The model under review builds one solid part; all positions refer to its coordinate system, in mm. A direction names the side the tool comes from. Give positions to 0.01 mm unless a question says otherwise; leave off trailing zeros. Order: outer loops, then holes, each group sorted by start corner. A loop starts at its lowest first (then second) coordinate and runs counter-clockwise, first axis right, second up. Notation, with made-up numbers: M 83,81 L 133,81 A23 ccw 133,93 Z; hole C 81.5,-4.75 d9. An arc over 180 degrees is marked long. One line per question, with ' | ' between items. Start each with the question number.
1. Wall thickness on L1, parallel to X at y = 9.5, z = -39; L2, parallel to Y at x = 36.5, z = -43.5; L3, parallel to X at y = 38, z = -23: over which ranges is each line inside the solid? List them lowest first.
2. We need section D-D on x = 38. Write out the cut boundary in (y, z), then the cut area to 3 significant figures.
3. Insertion check: P1, Ø10, axis at x = 13.5, y = 11, coming from the -Z side; P2, Ø8, axis at x = 14.5, y = 16, coming from the +Z side. Each pin has a flat end and moves straight along its axis. Give the tip position at first contact, or say it passes through.
4. We need section B-B on x = 23.5. Write out the cut boundary in (y, z).
5. The part is to be moulded in two halves that separate along X. For faces 4 (the face through (37.03, 18.24, -37.08)), 5 (the face through (9.92, 18.24, -37.03)), 6 (the face through (45.2, 20.7, -1.7)), 7 (the face through (18, 42, -34)), say which applies: +X half, -X half, draft (parallel to the pull), parting line (faces both ways), or undercut.
6. For faces 1 (the face through (23, 2, -8)), 2 (the face through (35.111, 21, -41)), 3 (the face through (37.65, 20.78, -44.54)), list the 3-axis set-ups (+Z, -Z, +X, -X, +Y, -Y) from which the entire face can be reached by the end or side of a thin tool; tool diameter is ignored.
7. We need section C-C on z = -23.5. Write out the cut boundary in (x, y).
8. We need section A-A on y = 27. Write out the cut boundary in (x, z), then the cut area to 3 significant figures.
```python
from build123d import *

# Parameters (mm, degrees)
SKETCH1_R           = 1.75
SKETCH1_W           = 8
SKETCH1_H           = 23.221825406
SKETCH1_W_2         = 23.221825406
SKETCH1_H_2         = 8
BOSS_EXTRUDE1_DEPTH = 5
SKETCH1_3_R         = 1.75
SKETCH1_3_W         = 8
SKETCH1_3_H         = 23.221825406
BOSS_EXTRUDE2_DEPTH = 42
BOSS_EXTRUDE3_START = 37
SKETCH1_4_R         = 11.5
SKETCH1_4_W         = 23.221825406
SKETCH1_4_H         = 8
SKETCH1_4_R_2       = 1.75
SKETCH1_4_W_2       = 8
SKETCH1_4_H_2       = 23.221825406
BOSS_EXTRUDE3_DEPTH = 5
CHAMFER2_SIZE       = 5
CHAMFER4_SIZE       = 3.5


with BuildPart() as part:
    # Sketch1 → Boss-Extrude1 (new body)
    # profile 1 of 8: a face of its own
    with BuildSketch(Plane(origin=(0, 0, 0), x_dir=(1, 0, 0), z_dir=(0, 1, 0))):
        Polygon((0, 47), (0, 35.110912703), (8, 35.110912703), (11.889087297, 39), (11.889087297, 47), align=None)
        with Locations(Location((8, 39, 0), (0, 0, 270))):
            Circle(SKETCH1_R, mode=Mode.SUBTRACT)
    # profile 2 of 8: a face of its own
    with BuildSketch(Plane(origin=(0, 0, 0), x_dir=(1, 0, 0), z_dir=(0, 1, 0))):
        with Locations((4, 23.5)):
            Rectangle(SKETCH1_W, SKETCH1_H)
    # profile 3 of 8: a face of its own
    with BuildSketch(Plane(origin=(0, 0, 0), x_dir=(1, 0, 0), z_dir=(0, 1, 0))):
        Polygon((0, 11.889087297), (0, 0), (11.889087297, 0), (11.889087297, 8), (8, 11.889087297), align=None)
        with Locations(Location((8, 8, 0), (0, 0, 270))):
            Circle(SKETCH1_R, mode=Mode.SUBTRACT)
    # profile 4 of 8: a face of its own
    with BuildSketch(Plane(origin=(0, 0, 0), x_dir=(1, 0, 0), z_dir=(0, 1, 0))):
        with Locations((23.5, 4)):
            Rectangle(SKETCH1_W_2, SKETCH1_H_2)
    # profile 5 of 8: a face of its own
    with BuildSketch(Plane(origin=(0, 0, 0), x_dir=(1, 0, 0), z_dir=(0, 1, 0))):
        Polygon((35.110912703, 8), (35.110912703, 0), (47, 0), (47, 11.889087297), (39, 11.889087297), align=None)
        with Locations(Location((39, 8, 0), (0, 0, 270))):
            Circle(SKETCH1_R, mode=Mode.SUBTRACT)
    # profile 6 of 8: a face of its own
    with BuildSketch(Plane(origin=(0, 0, 0), x_dir=(1, 0, 0), z_dir=(0, 1, 0))):
        with Locations((43, 23.5)):
            Rectangle(SKETCH1_W, SKETCH1_H)
    # profile 7 of 8: a face of its own
    with BuildSketch(Plane(origin=(0, 0, 0), x_dir=(1, 0, 0), z_dir=(0, 1, 0))):
        Polygon((39, 35.110912703), (47, 35.110912703), (47, 47), (35.110912703, 47), (35.110912703, 39), align=None)
        with Locations(Location((39, 39, 0), (0, 0, 270))):
            Circle(SKETCH1_R, mode=Mode.SUBTRACT)
    # profile 8 of 8: a face of its own
    with BuildSketch(Plane(origin=(0, 0, 0), x_dir=(1, 0, 0), z_dir=(0, 1, 0))):
        with Locations((23.5, 43)):
            Rectangle(SKETCH1_W_2, SKETCH1_H_2)
    extrude(amount=BOSS_EXTRUDE1_DEPTH)

    # Sketch1<3> → Boss-Extrude2 (add)
    # profile 1 of 6: a face of its own
    with BuildSketch(Plane(origin=(0, 0, 0), x_dir=(1, 0, 0), z_dir=(0, 1, 0))):
        Polygon((0, 11.889087297), (0, 0), (11.889087297, 0), (11.889087297, 8), (8, 11.889087297), align=None)
        with Locations(Location((8, 8, 0), (0, 0, 270))):
            Circle(SKETCH1_3_R, mode=Mode.SUBTRACT)
    # profile 2 of 6: a face of its own
    with BuildSketch(Plane(origin=(0, 0, 0), x_dir=(1, 0, 0), z_dir=(0, 1, 0))):
        Polygon((0, 47), (0, 35.110912703), (8, 35.110912703), (11.889087297, 39), (11.889087297, 47), align=None)
        with Locations(Location((8, 39, 0), (0, 0, 270))):
            Circle(SKETCH1_3_R, mode=Mode.SUBTRACT)
    # profile 3 of 6: a face of its own
    with BuildSketch(Plane(origin=(0, 0, 0), x_dir=(1, 0, 0), z_dir=(0, 1, 0))):
        Polygon((39, 35.110912703), (47, 35.110912703), (47, 47), (35.110912703, 47), (35.110912703, 39), align=None)
        with Locations(Location((39, 39, 0), (0, 0, 270))):
            Circle(SKETCH1_3_R, mode=Mode.SUBTRACT)
    # profile 4 of 6: a face of its own
    with BuildSketch(Plane(origin=(0, 0, 0), x_dir=(1, 0, 0), z_dir=(0, 1, 0))):
        Polygon((35.110912703, 8), (35.110912703, 0), (47, 0), (47, 11.889087297), (39, 11.889087297), align=None)
        with Locations(Location((39, 8, 0), (0, 0, 270))):
            Circle(SKETCH1_3_R, mode=Mode.SUBTRACT)
    # profile 5 of 6: a face of its own
    with BuildSketch(Plane(origin=(0, 0, 0), x_dir=(1, 0, 0), z_dir=(0, 1, 0))):
        with Locations((4, 23.5)):
            Rectangle(SKETCH1_3_W, SKETCH1_3_H)
    # profile 6 of 6: a face of its own
    with BuildSketch(Plane(origin=(0, 0, 0), x_dir=(1, 0, 0), z_dir=(0, 1, 0))):
        with Locations((43, 23.5)):
            Rectangle(SKETCH1_3_W, SKETCH1_3_H)
    extrude(amount=BOSS_EXTRUDE2_DEPTH)

    # Sketch1<4> → Boss-Extrude3 (add)
    # profile 1 of 9: a face of its own
    with BuildSketch(Plane(origin=(0, 0, 0), x_dir=(1, 0, 0), z_dir=(0, 1, 0)).offset(BOSS_EXTRUDE3_START)):
        Polygon((11.889087297, 39), (8, 35.110912703), (8, 11.889087297), (11.889087297, 8), (35.110912703, 8), (39, 11.889087297), (39, 35.110912703), (35.110912703, 39), align=None)
        with Locations(Location((23.5, 23.5, 0), (0, 0, 270))):
            Circle(SKETCH1_4_R, mode=Mode.SUBTRACT)
    # profile 2 of 9: a face of its own
    with BuildSketch(Plane(origin=(0, 0, 0), x_dir=(1, 0, 0), z_dir=(0, 1, 0)).offset(BOSS_EXTRUDE3_START)):
        with Locations((23.5, 43)):
            Rectangle(SKETCH1_4_W, SKETCH1_4_H)
    # profile 3 of 9: a face of its own
    with BuildSketch(Plane(origin=(0, 0, 0), x_dir=(1, 0, 0), z_dir=(0, 1, 0)).offset(BOSS_EXTRUDE3_START)):
        Polygon((0, 47), (0, 35.110912703), (8, 35.110912703), (11.889087297, 39), (11.889087297, 47), align=None)
        with Locations(Location((8, 39, 0), (0, 0, 270))):
            Circle(SKETCH1_4_R_2, mode=Mode.SUBTRACT)
    # profile 4 of 9: a face of its own
    with BuildSketch(Plane(origin=(0, 0, 0), x_dir=(1, 0, 0), z_dir=(0, 1, 0)).offset(BOSS_EXTRUDE3_START)):
        with Locations((4, 23.5)):
            Rectangle(SKETCH1_4_W_2, SKETCH1_4_H_2)
    # profile 5 of 9: a face of its own
    with BuildSketch(Plane(origin=(0, 0, 0), x_dir=(1, 0, 0), z_dir=(0, 1, 0)).offset(BOSS_EXTRUDE3_START)):
        Polygon((0, 11.889087297), (0, 0), (11.889087297, 0), (11.889087297, 8), (8, 11.889087297), align=None)
        with Locations(Location((8, 8, 0), (0, 0, 270))):
            Circle(SKETCH1_4_R_2, mode=Mode.SUBTRACT)
    # profile 6 of 9: a face of its own
    with BuildSketch(Plane(origin=(0, 0, 0), x_dir=(1, 0, 0), z_dir=(0, 1, 0)).offset(BOSS_EXTRUDE3_START)):
        with Locations((23.5, 4)):
            Rectangle(SKETCH1_4_W, SKETCH1_4_H)
    # profile 7 of 9: a face of its own
    with BuildSketch(Plane(origin=(0, 0, 0), x_dir=(1, 0, 0), z_dir=(0, 1, 0)).offset(BOSS_EXTRUDE3_START)):
        Polygon((35.110912703, 8), (35.110912703, 0), (47, 0), (47, 11.889087297), (39, 11.889087297), align=None)
        with Locations(Location((39, 8, 0), (0, 0, 270))):
            Circle(SKETCH1_4_R_2, mode=Mode.SUBTRACT)
    # profile 8 of 9: a face of its own
    with BuildSketch(Plane(origin=(0, 0, 0), x_dir=(1, 0, 0), z_dir=(0, 1, 0)).offset(BOSS_EXTRUDE3_START)):
        with Locations((43, 23.5)):
            Rectangle(SKETCH1_4_W_2, SKETCH1_4_H_2)
    # profile 9 of 9: a face of its own
    with BuildSketch(Plane(origin=(0, 0, 0), x_dir=(1, 0, 0), z_dir=(0, 1, 0)).offset(BOSS_EXTRUDE3_START)):
        Polygon((39, 35.110912703), (47, 35.110912703), (47, 47), (35.110912703, 47), (35.110912703, 39), align=None)
        with Locations(Location((39, 39, 0), (0, 0, 270))):
            Circle(SKETCH1_4_R_2, mode=Mode.SUBTRACT)
    extrude(amount=BOSS_EXTRUDE3_DEPTH)

    # Chamfer2
    chamfer2_edges = [part.edges().sort_by_distance(p)[0] for p in [
        (35.110912703, 21, -47),
        (35.110912703, 21, 0),
        (11.889087297, 21, 0),
        (11.889087297, 21, -47),
    ]]
    chamfer(chamfer2_edges, length=CHAMFER2_SIZE)

    # Chamfer4
    chamfer4_edges = [part.edges().sort_by_distance(p)[0] for p in [
        (0, 21, 0),
        (0, 21, -47),
        (47, 21, -47),
        (47, 21, 0),
    ]]
    chamfer(chamfer4_edges, length=CHAMFER4_SIZE)


solid = part.part
```
Entries:
1) L1: x = 0 to 6.25, 9.75 to 11.89, 35.11 to 37.25, 40.75 to 47 | L2: y = 0 to 5, 37 to 42 | L3: x = 0 to 12.01, 34.99 to 47
2) outline: M 0,-47 L 5,-47 L 5,-44.89 L 37,-44.89 L 37,-47 L 42,-47 L 42,-40.44 L 0,-40.44 Z; M 0,-37.56 L 42,-37.56 L 42,-9.44 L 0,-9.44 L 0,-10.89 L 37,-10.89 L 37,-36.11 L 0,-36.11 Z; M 0,-6.56 L 42,-6.56 L 42,0 L 37,0 L 37,-2.11 L 5,-2.11 L 5,0 L 0,0 Z | area: 664 mm^2
3) P1: stops at z = -45.39 | P2: stops at z = -3.61
4) outline: M 0,-47 L 5,-47 L 5,-39 L 0,-39 Z; M 0,-8 L 5,-8 L 5,0 L 0,0 Z; M 37,-47 L 42,-47 L 42,-35 L 37,-35 Z; M 37,-12 L 42,-12 L 42,0 L 37,0 Z
5) face 4: undercut | face 5: undercut | face 6: +X half | face 7: draft
6) face 1: -Y | face 2: +Z, -Z | face 3: -Z
7) outline: M 0,0 L 8,0 L 8,37 L 12,37 L 12,42 L 0,42 Z; M 35,37 L 39,37 L 39,0 L 47,0 L 47,42 L 35,42 Z
8) outline: M 0,-43.5 L 3.5,-47 L 6.89,-47 L 11.89,-42 L 11.89,-39 L 8,-35.11 L 8,-11.89 L 11.89,-8 L 11.89,-5 L 6.89,0 L 3.5,0 L 0,-3.5 Z; M 35.11,-42 L 40.11,-47 L 43.5,-47 L 47,-43.5 L 47,-3.5 L 43.5,0 L 40.11,0 L 35.11,-5 L 35.11,-8 L 39,-11.89 L 39,-35.11 L 35.11,-39 Z; hole C 8,-39 d3.5; hole C 8,-8 d3.5; hole C 39,-39 d3.5; hole C 39,-8 d3.5 | area: 794 mm^2
